CAD build for the part. Positions are in the model's coordinates, mm. Coordinates: 2 decimals unless noted, no trailing zeros. Write each loop counter-clockwise with the first axis right and the second up, starting at its lowest first coordinate (ties: lowest second). Pieces come first, ordered by that corner, then holes.
```python
from build123d import *

# Parameters (mm, degrees)
SKETCH1_R           = 3.302
BOSS_EXTRUDE1_DEPTH = 3.175
FILLET6_R           = 35.56
FILLET10_R          = 27.94
FILLET13_R          = 50.8
FILLET16_R          = 20.32


with BuildPart() as part:
    # Sketch1 → Boss-Extrude1 (new body)
    with BuildSketch(Plane(origin=(0, 0, 0), x_dir=(-1, 0, 0), z_dir=(0, 0, -1))):
        with BuildLine():
            Line((165.785053206, 142.946766421), (130.990896358, 174.574150067))
            Line((130.990896358, 174.574150067), (31.981087973, 112.057039535))
            Line((31.981087973, 112.057039535), (9.409224511, 1.710371233))
            ThreePointArc((9.409224511, 1.710371233), (21.197749586, -18.801775256), (43.01064713, -9.641263383))
            Line((43.01064713, -9.641263383), (77.484953862, 85.860414024))
            Line((77.484953862, 85.860414024), (165.785053206, 142.946766421))
        make_face()
        with Locations((32.554001794, 24.213373462)):
            Circle(SKETCH1_R, mode=Mode.SUBTRACT)
        with Locations((94.707078764, 129.476886965)):
            Circle(SKETCH1_R, mode=Mode.SUBTRACT)
    extrude(amount=-BOSS_EXTRUDE1_DEPTH)

    # Fillet6
    fillet6_edges = [part.edges().sort_by_distance(p)[0] for p in [
        (-130.990896358, 174.574150067, 1.5875),
    ]]
    fillet(fillet6_edges, radius=FILLET6_R)

    # Fillet10
    fillet10_edges = [part.edges().sort_by_distance(p)[0] for p in [
        (-31.981087973, 112.057039535, 1.5875),
    ]]
    fillet(fillet10_edges, radius=FILLET10_R)

    # Fillet13
    fillet13_edges = [part.edges().sort_by_distance(p)[0] for p in [
        (-77.484953862, 85.860414024, 1.5875),
    ]]
    fillet(fillet13_edges, radius=FILLET13_R)

    # Fillet16
    fillet16_edges = [part.edges().sort_by_distance(p)[0] for p in [
        (-165.785053206, 142.946766421, 1.5875),
    ]]
    fillet(fillet16_edges, radius=FILLET16_R)


solid = part.part
```
Item 1: Two-plate mould, pull along X, no slides. Class faces 1 (the cylindrical face through (-93.991, 126.253, 1.565)), 2 (the flat face through (-63, 74, 3.175)), 3 (the cylindrical face through (-20.9, -18.7, 1.6)), 4 (the flat face through (-75.54, 139.56, 1.57)): +X half, -X half, draft (parallel to the pull), parting line (faces both ways), or undercut.
Item 2: Saw through at A-A, the plane y = -6. Write the cut outline in (x, z) (3 decimals), and give its area (3 significant figures).
Item 3: Saw through at C-C, the plane z = 1.9. State how many separate pieces and enclosed holes the cut face has, and give its area (3 significant figures).
Item 4: Wall check: line 1 along Y through (x, z) = (-93.5, 1); line 2 along Y through (x, z) = (-132.5, 2.8); line 3 along Y through (x, z) = (-108, 0.45). Give the ranges that are in metal, low to high.
Item 5: Flat gauge pins, fed straight in: pin 1 Ø10 at (x, y) = (-109, 145) entering from -Z; pin 2 Ø1 at (y, z) = (28, 1) entering from +X. Where does each tip first touch, or does it go through?
Item 6: Saw through at B-B, the plane x = -18. Write the cut outline in (y, z) (3 decimals), and give its area (3 significant figures).
Working result:
1. face 1: undercut
1. face 2: draft
1. face 3: parting line
1. face 4: +X half
2. outline: (-44.325, 0) - (-9.53, 0) - (-9.53, 3.175) - (-44.325, 3.175) - close
2. area: 110 mm2
3. separate pieces: 1
3. enclosed holes: 2
3. area: 9,740 mm2
4. line 1: y = 96.21 to 126.4, 132.55 to 150.9
4. line 2: y = 121.43 to 165.21
4. line 3: y = 105.59 to 160.06
5. pin 1: stops at z = 0
5. pin 2: stops at x = -14.68
6. outline: (-17.358, 0) - (43.708, 0) - (43.708, 3.175) - (-17.358, 3.175) - close
6. area: 194 mm2
